Can you work these out from the drawing? Everything is in mm from the part's minimum corner. A direction names the side the tool comes from. Round coordinates to 2 decimals unless told otherwise and drop trailing zeros. Order: outer loops, then holes, each group sorted by start corner. A loop starts at its lowest first (then second) coordinate and runs counter-clockwise, first axis right, second up. Notation, with made-up numbers: (11.25, 17) - (29.25, 17) arc R24 ccw to (29.25, 28) - close; hole circle Ø6 at (-19.5, 1.5). An arc over 180 degrees is marked (long way). Answer as a JSON object with one key per item and string values.
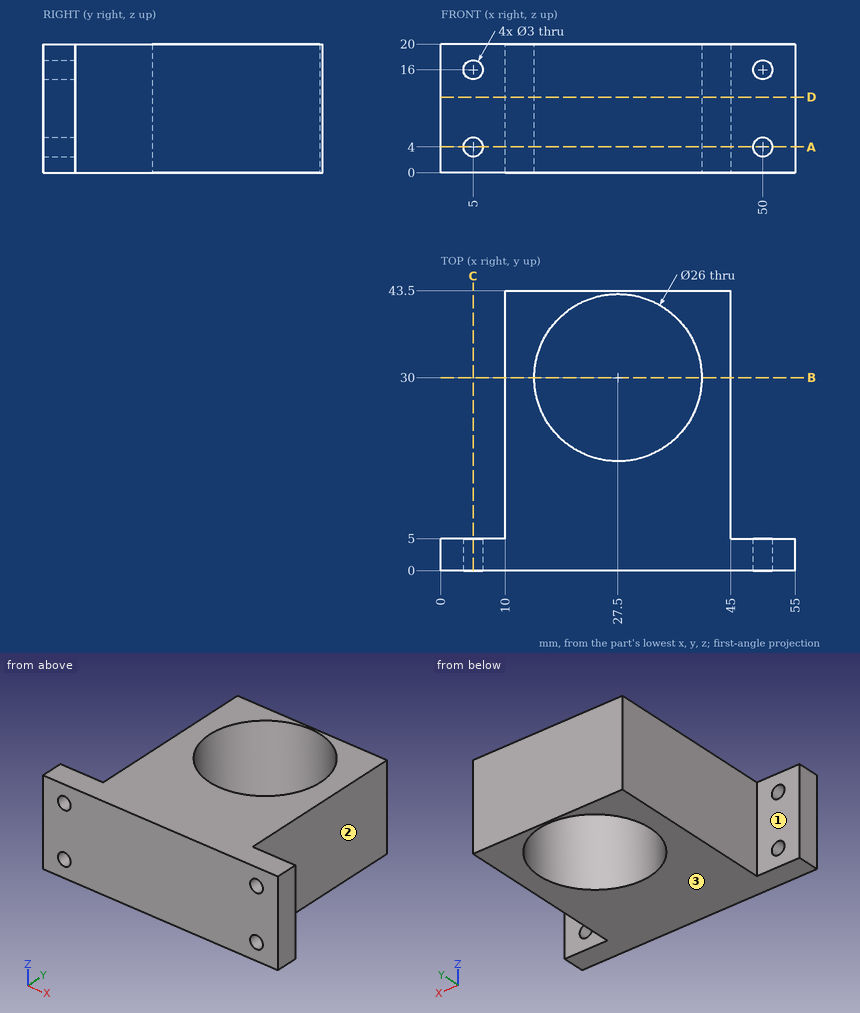
1. Imagine slicing it at D-D (z = 11.75). List the corners of the cut face in (x, y) for me, plus the area to 3 significant figures.
Responses:
{"outline": "(0, 0) - (55, 0) - (55, 5) - (45, 5) - (45, 43.5) - (10, 43.5) - (10, 5) - (0, 5) - close; hole circle Ø26 at (27.5, 30)", "area": "1,090 mm2"}
2. Imagine slicing it at A-A (z = 4). List the corners of the cut face in (x, y) for me.
Responses:
{"outline": "(0, 0) - (3.5, 0) - (3.5, 5) - (0, 5) - close; (6.5, 0) - (48.5, 0) - (48.5, 5) - (45, 5) - (45, 43.5) - (10, 43.5) - (10, 5) - (6.5, 5) - close; (51.5, 0) - (55, 0) - (55, 5) - (51.5, 5) - close; hole circle Ø26 at (27.5, 30)"}
3. For P1, Ø6, axis at y = 23, z = 10.5, coming from the +X side; P2, Ø1, axis at y = 14.5, z = 17, coming from the -X side; P3, Ø5, axis at x = 7, z = 5, coming from the +Y side; P4, Ø2, axis at x = 19, z = 13.5, coming from the -Y side, each with a flat end and sliding along its axis, tell me the tip position at first contact or that it passes through.
Responses:
{"P1": "x = 45", "P2": "x = 10", "P3": "y = 5", "P4": "y = 0"}
4. If I drill on L1, parallel to Z at x = 5, y = 1; L2, parallel to X at y = 1.7, z = 4; L3, parallel to X at y = 29.5, z = 18.5, over which ranges is the centre line in solid material (lowest first)? Write a range as [from, to].
Responses:
{"L1": "[0, 2.5], [5.5, 14.5], [17.5, 20]", "L2": "[0, 3.5], [6.5, 48.5], [51.5, 55]", "L3": "[10, 14.51], [40.49, 45]"}
5. Imagine slicing it at C-C (x = 5). List the corners of the cut face in (y, z) for me, plus the area to 3 significant figures.
Responses:
{"outline": "(0, 0) - (5, 0) - (5, 2.5) - (0, 2.5) - close; (0, 5.5) - (5, 5.5) - (5, 14.5) - (0, 14.5) - close; (0, 17.5) - (5, 17.5) - (5, 20) - (0, 20) - close", "area": "70.0 mm2"}
6. Imagine slicing it at B-B (y = 30). List the corners of the cut face in (x, z) for me, plus the area to 3 significant figures.
Responses:
{"outline": "(10, 0) - (14.5, 0) - (14.5, 20) - (10, 20) - close; (40.5, 0) - (45, 0) - (45, 20) - (40.5, 20) - close", "area": "180 mm2"}
7. For the marked faces 1, 2 and 3, which set-ups out of +Z, -Z, +X, -X, +Y, -Y let a thin tool reach every point of the face, with its end or its side?
Responses:
{"face 1": "+Z, -Z, -X, +Y", "face 2": "+Z, -Z, +X, +Y", "face 3": "-Z, +X, -X, +Y, -Y"}
